```python
from build123d import *

# Parameters (mm, degrees)
REVOLVE1_ANGLE = 10


with BuildPart() as part:
    # Sketch1 → Revolve1 (revolve)
    with BuildSketch(Plane(origin=(0, 0, 0), x_dir=(1, 0, 0), z_dir=(0, 1, 0))):
        with BuildLine():
            Line((75, 190.7), (83, 190.7))
            Line((83, 190.7), (83, 129.833691726))
            ThreePointArc((83, 129.833691726), (142.120054058, 59.562385293), (150.766644537, -31.862303784))
            Line((150.766644537, -31.862303784), (147.766644537, -31.862303784))
            ThreePointArc((147.766644537, -31.862303784), (138.047901954, 61.587047389), (75, 131.244762334))
            Line((75, 131.244762334), (75, 190.7))
        make_face()
    revolve(axis=Axis((0, 0, 125), (0, 0, -1)), revolution_arc=REVOLVE1_ANGLE)


solid = part.part
```
For this review, take the finished solid that the model builds, in its own axes (mm). A direction names the side the tool comes from. Round coordinates to 2 decimals unless told otherwise and drop trailing zeros. Order: outer loops, then holes, each group sorted by start corner. A loop starts at its lowest first (then second) coordinate and runs counter-clockwise, first axis right, second up. Notation, with made-up numbers: (35.5, 86) -> (82.5, 86) arc R12 cw to (82.5, 100) -> close; hole circle Ø9 at (59, 3). An arc over 180 degrees is marked (long way). Use a Markdown table: item, result.
Item 1: Take a section at C-C (x = 121). State the section outline as (y, z) points.
Resolved:
| item | result |
|---|---|
| outline | (-21.34, -93) arc R95.42 ccw to (0, -95.42) -> (0, -90.6) arc R90.6 cw to (-21.34, -88.06) -> close |
Item 2: Machinability: for faces 1 (the cylindrical face through (82.693, -7.133, -159.841)), 2 (the flat face through (149, -13, 31.862)), which of the approach directions +Z, -Z, +X, -X, +Y, -Y give a long, thin tool a straight path to every point of the face, cutting with its end or side? Answer none if there is none.
Resolved:
| item | result |
|---|---|
| face 1 | -Z, +X, -Y |
| face 2 | +Z, +X, -X, +Y, -Y |
Item 3: For pin 1 (5 mm diameter, centred on x = 126.5, y = -17.5, fed in from +Z); pin 2 (6 mm diameter, centred on x = 100.5, y = -17.5, fed in from -Z); pin 3 (4 mm diameter, centred on y = -20.5, z = -28.5, fed in from +X), all flat-tipped, find the tip position at first contact; note any pin that passes through.
Resolved:
| item | result |
|---|---|
| pin 1 | stops at z = -76.79 |
| pin 2 | stops at z = -118.08 |
| pin 3 | stops at x = 150.5 |
Item 4: Take a section at A-A (y = -11). State the section outline as (x, z) points.
Resolved:
| item | result |
|---|---|
| outline | (74.19, -190.7) -> (82.27, -190.7) -> (82.27, -129.83) arc R153.7 ccw to (150.36, 31.86) -> (147.36, 31.86) arc R150.76 cw to (74.19, -131.24) -> close |
Item 5: For line 1 along X through (y, z) = (-4.75, -14); line 2 along Z through (x, y) = (114.5, -7.75); line 3 along X through (y, z) = (-14, -100), list the stretches that pass through material, from the lowest coordinate up. Write a range as [from, to].
Resolved:
| item | result |
|---|---|
| line 1 | x = [150.44, 153.39] |
| line 2 | z = [-102.84, -98.39] |
| line 3 | x = [112.49, 116.4] |
Item 6: Take a section at B-B (z = -134). State the section outline as (x, y) points.
Resolved:
| item | result |
|---|---|
| outline | (73.86, -13.02) -> (81.74, -14.41) arc R83 ccw to (83, 0) -> (75, 0) arc R75 cw to start |
